For this review, take the finished solid that the model builds, in its own axes (mm). Face numbers are marked on the shaded views. A direction names the side the tool comes from. Give positions to 0.01 mm unless a question says otherwise; leave off trailing zeros. Write each loop counter-clockwise with the first axis right and the second up, starting at its lowest first coordinate (ties: lowest second). Pieces come first, ordered by that corner, then holes. Notation, with made-up numbers: (39, -25.5) -> (61, -25.5) arc R19 cw to (61, 11.5) -> close; hole circle Ø1 at (68.25, 69). An arc over 180 degrees is marked (long way). Return JSON: item names as keys, results as strings.
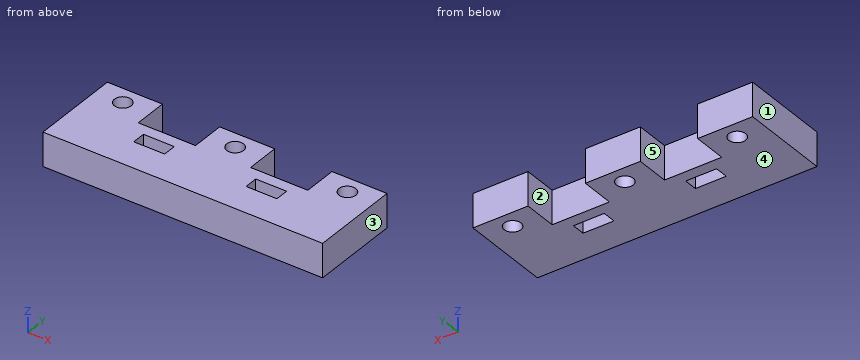
Autodesk Inventor part; units mm, degrees
ref_plane "YZ Plane" through (0, 0, 0) normal (1, 0, 0) x (0, 1, 0)
ref_plane "XZ Plane" through (0, 0, 0) normal (0, 1, 0) x (-1, 0, 0)
ref_plane "XY Plane" through (0, 0, 0) normal (0, 0, 1) x (1, 0, 0)
sketch "Sketch1" plane through (0, 0, 0) normal (0, 0, 1) x (1, 0, 0)
  line L0 (0, 0) -> (9.8, 0)
  line L1 (9.8, 0) -> (9.8, 6)
  line L2 (9.8, 6) -> (0, 6)
  line L3 (0, 6) -> (0, 0)
  line L4 (29.8, 6) -> (20, 6)
  line L5 (20, 6) -> (20, 0)
  line L6 (20, 0) -> (29.8, 0)
  line L7 (29.8, 0) -> (29.8, 6)
  line L8 (49.8, 6) -> (40, 6)
  line L9 (40, 6) -> (40, 0)
  line L10 (40, 0) -> (49.8, 0)
  line L11 (49.8, 0) -> (49.8, 6)
  circle A0 centre (4.9, 3) radius 1.5
  circle A1 centre (24.9, 3) radius 1.5
  circle A2 centre (44.9, 3) radius 1.5
  line L12 (0, 0) -> (49.8, 0)
  line L13 (49.8, 0) -> (49.8, -10)
  line L14 (49.8, -10) -> (0, -10)
  line L15 (0, -10) -> (0, 0)
  line L16 (12.15, -2) -> (17.65, -2)
  line L17 (17.65, -2) -> (17.65, -4.4)
  line L18 (17.65, -4.4) -> (12.15, -4.4)
  line L19 (12.15, -4.4) -> (12.15, -2)
  line L20 (32.15, -2) -> (37.65, -2)
  line L21 (37.65, -2) -> (37.65, -4.4)
  line L22 (37.65, -4.4) -> (32.15, -4.4)
  line L23 (32.15, -4.4) -> (32.15, -2)
  point P0 (40, 0)
  point P1 (20, 0)
  dimension "d0" = 6
  dimension "d1" = 9.8
  dimension "d4" = 20
  dimension "d9" = 3
  dimension "d12" = 20
  dimension "d17" = 10
  dimension "d20" = 5.5
  dimension "d21" = 2.4
  dimension "d22" = 2.35
  dimension "d23" = 8
  dimension "d24" = 3
  dimension "d27" = 20
extrude "Extrusion1" add sketch "Sketch1" along normal blind 6
properties part number "SideBoardTest"
1. Add section B-B, the plane x = 14. State the section outline as (y, z) points.
Results found:
{"outline": "(-10, 0) -> (-4.4, 0) -> (-4.4, 6) -> (-10, 6) -> close; (-2, 0) -> (0, 0) -> (0, 6) -> (-2, 6) -> close"}
2. To check wall thickness, follow probe 1 along Y at (x, z) = (15, 5.65); probe 2 along Y at (x, z) = (44.9, 4.25); probe 3 along X at (y, z) = (2, 2.45). State the ranges of each line that lie inside material, in increasing order.
Results found:
{"probe 1": "y = -10 to -4.4, -2 to 0", "probe 2": "y = -10 to 1.5, 4.5 to 6", "probe 3": "x = 0 to 3.78, 6.02 to 9.8, 20 to 23.78, 26.02 to 29.8, 40 to 43.78, 46.02 to 49.8"}
3. Add section D-D, the plane x = 4.9. State the section outline as (y, z) points.
Results found:
{"outline": "(-10, 0) -> (1.5, 0) -> (1.5, 6) -> (-10, 6) -> close; (4.5, 0) -> (6, 0) -> (6, 6) -> (4.5, 6) -> close"}
4. The part is to be moulded in two halves that separate along X. For the marked faces 3, 4 and 5, say which applies: +X half, -X half, draft (parallel to the pull), parting line (faces both ways), or undercut.
Results found:
{"face 3": "+X half", "face 4": "draft", "face 5": "undercut"}
5. Add section C-C, the plane z = 1.4. State the section outline as (x, y) points, plus the area to 3 significant figures.
Results found:
{"outline": "(0, -10) -> (49.8, -10) -> (49.8, 6) -> (40, 6) -> (40, 0) -> (29.8, 0) -> (29.8, 6) -> (20, 6) -> (20, 0) -> (9.8, 0) -> (9.8, 6) -> (0, 6) -> close; hole circle Ø3 at (4.9, 3); hole (12.15, -4.4) -> (17.65, -4.4) -> (17.65, -2) -> (12.15, -2) -> close; hole circle Ø3 at (24.9, 3); hole (32.15, -4.4) -> (37.65, -4.4) -> (37.65, -2) -> (32.15, -2) -> close; hole circle Ø3 at (44.9, 3)", "area": "627 mm²"}
6. For the marked faces 1 and 2, list the 3-axis set-ups (+Z, -Z, +X, -X, +Y, -Y) from which the entire face can be reached by the end or side of a thin tool; tool diameter is ignored.
Results found:
{"face 1": "+Z, -Z, -X, +Y, -Y", "face 2": "+Z, -Z, +Y"}
7. For pin 1 (3 mm diameter, centred on x = 15.5, z = 2, fed in from +Y), flat-tipped, find the tip position at first contact; note if it passes through.
Results found:
{"pin 1": "stops at y = 0"}
8. Add section A-A, the plane y = 1. State the section outline as (x, z) points.
Results found:
{"outline": "(0, 0) -> (9.8, 0) -> (9.8, 6) -> (0, 6) -> close; (20, 0) -> (29.8, 0) -> (29.8, 6) -> (20, 6) -> close; (40, 0) -> (49.8, 0) -> (49.8, 6) -> (40, 6) -> close"}
